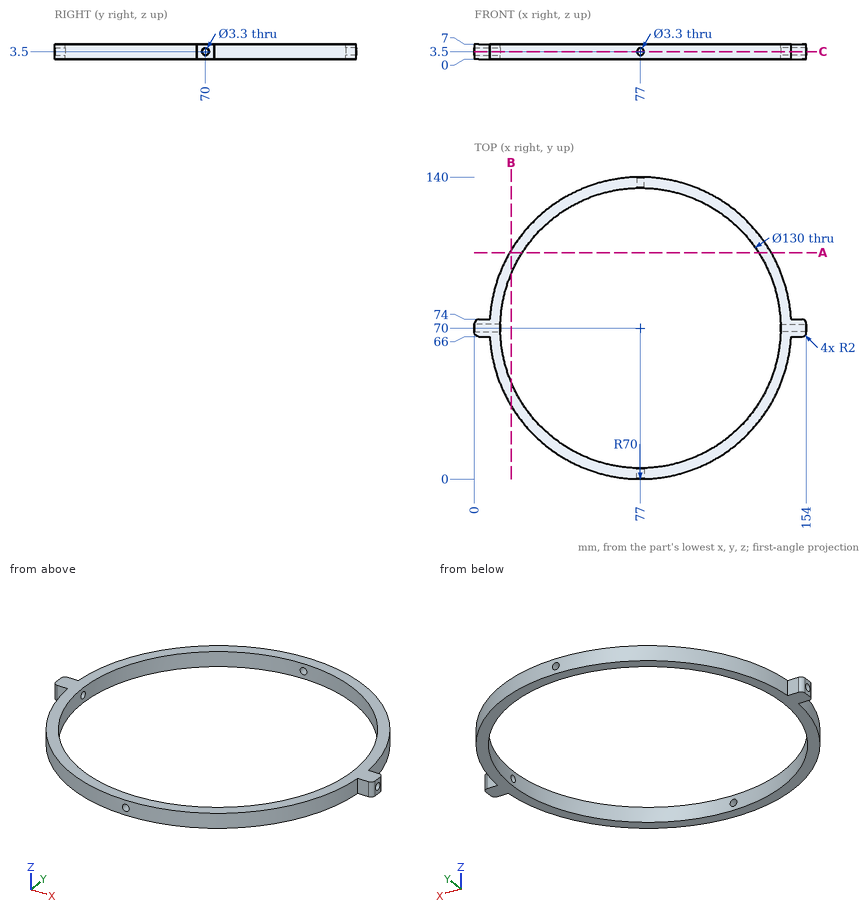
Print and shaded views of the part. All mm, measured from the part's lowest x, y and z. Coordinates: 2 decimals unless noted, no trailing zeros. Loops run counter-clockwise (first coordinate to the right, second up) from the corner with the lowest first, then second, coordinate; pieces in that order, holes last. Notation, with made-up numbers: (-24.75, 74) -> (9.25, 74) arc R24 cw to (9.25, 103) -> close; hole circle Ø2 at (-3.75, 88.5). An arc over 180 degrees is marked (long way). Use a Markdown table: item, result. Add a question column.
Item 1: Band-saw the part on B-B on x = 17. Write the cut outline in (y, z), plus the area to 3 significant figures.
Item 2: Flat gauge pins, fed straight in: P1, Ø4, axis at x = 3.5, z = 3.5, coming from the +Y side; P2, Ø4, axis at x = 149, z = 3, coming from the -Y side; P3, Ø4, axis at y = 70, z = 3.5, coming from the +X side. Where does each tip first touch, or does it go through?
Item 3: Band-saw the part on A-A on y = 105. Write the cut outline in (x, z).
Item 4: Probe probe 1 along Z at (x, y) = (146.75, 70); probe 2 along X at (y, z) = (86, 1.5); probe 3 along X at (y, z) = (103.5, 3.75). List the from-to ranges inside material, lowest first.
Item 5: Band-saw the part on C-C on z = 3.5. Write the cut outline in (x, y).
Geometry says:
| question | item | result |
|---|---|---|
| 1 | outline | (33.94, 0) -> (45, 0) -> (45, 7) -> (33.94, 7) -> close; (95, 0) -> (106.06, 0) -> (106.06, 7) -> (95, 7) -> close |
| 1 | area | 155 mm² |
| 2 | P1 | y = 74 |
| 2 | P2 | y = 66 |
| 2 | P3 | x = 154 |
| 3 | outline | (16.38, 0) -> (22.23, 0) -> (22.23, 7) -> (16.38, 7) -> close; (131.77, 0) -> (137.62, 0) -> (137.62, 7) -> (131.77, 7) -> close |
| 4 | probe 1 | 0 to 1.85, 5.15 to 7 |
| 4 | probe 2 | 8.85 to 14, 140 to 145.15 |
| 4 | probe 3 | 15.54 to 21.3, 132.7 to 138.46 |
| 5 | outline | (0, 68) arc R2 ccw to (2, 66) -> (7.11, 66) arc R70 ccw to (75.35, 0.02) -> (75.35, 5.02) arc R65 cw to (12.02, 68.35) -> (0, 68.35) -> close; (0, 71.65) -> (12.02, 71.65) arc R65 cw to (75.35, 134.98) -> (75.35, 139.98) arc R70 ccw to (7.11, 74) -> (2, 74) arc R2 ccw to (0, 72) -> close; (78.65, 0.02) arc R70 ccw to (146.89, 66) -> (152, 66) arc R2 ccw to (154, 68) -> (154, 68.35) -> (141.98, 68.35) arc R65 cw to (78.65, 5.02) -> close; (78.65, 134.98) arc R65 cw to (141.98, 71.65) -> (154, 71.65) -> (154, 72) arc R2 ccw to (152, 74) -> (146.89, 74) arc R70 ccw to (78.65, 139.98) -> close |
